Check sheet for the modelled part. Datum: model origin and axes. Units: mm. A direction names the side the tool comes from. Coordinates: 2 decimals unless noted, no trailing zeros. Write each loop counter-clockwise with the first axis right and the second up, starting at its lowest first coordinate (ties: lowest second). Pieces come first, ordered by that corner, then holes. Notation, with made-up numbers: M 60,88 L 117,88 A28 ccw 117,113 Z; hole C 30,64.25 d11. An arc over 180 degrees is marked long. Answer as CSV lines item,"result". Start each with the question number.
1) Section check B-B (y = 63). Record the cut outline in (x, z), and give its area (3 significant figures).
2) Material ranges on L1, parallel to Y at x = 135, z = 45; L2, parallel to Z at x = 498.5, y = -60, recorded low to high. Write a range as [from, to].
3) Access from +Z, -Z, +X, -X, +Y, -Y to the whole of each face (thin tool, end or side, straight path). Record for faces 1 (the flat face through (10, -140, 55)), 2 (the flat face through (-10, 6, 3)).
4) Section check A-A (x = 340.5). Record the cut outline in (y, z), and give its area (3 significant figures).
5) Section check C-C (z = 64.5). Record the cut outline in (x, y), and give its area (3 significant figures).
6) Go/stop test with flat-tipped pins: pin 1 Ø12 at (x, z) = (354, 64) entering from +Y; pin 2 Ø6 at (x, y) = (179.5, -69) entering from +Z. Record where each tip stops, or that it passes through.
Autodesk Inventor part; units mm, degrees
ref_plane "YZ Plane" through (0, 0, 0) normal (1, 0, 0) x (0, 1, 0)
ref_plane "XZ Plane" through (0, 0, 0) normal (0, 1, 0) x (-1, 0, 0)
ref_plane "XY Plane" through (0, 0, 0) normal (0, 0, 1) x (1, 0, 0)
sketch "Sketch1" plane through (0, 0, 0) normal (0, 0, 1) x (1, 0, 0)
  line L0 (700, 140) -> (-700, 140)
  line L1 (-700, 140) -> (-700, -140)
  line L2 (-700, -140) -> (700, -140)
  line L3 (700, -140) -> (700, 140)
  line L4 (700, 140) -> (-700, -140) construction
  line L5 (-700, 140) -> (700, -140) construction
  point P0 (0, 0)
  point P1 (0, 0)
  point P2 (700, 0)
  dimension "d32" = 280
  dimension "d33" = 1400
extrude "Plate1" add sketch "Sketch1" along normal blind 3
sketch "Sketch6" plane through (700, -137, 0) normal (0, -1, 0) x (1, 0, 0)
  line L0 (-1400, 0) -> (0, 0)
  line L1 (0, 0) -> (0, 100)
  line L2 (0, 100) -> (-1400, 100)
  line L3 (-1400, 100) -> (-1400, 0)
edge flange "Flange2" height 100 angle 90 thickness 3 bend radius 5 thickness toward (0, -1, 0) relief round relief width 3 relief depth 1.5 edges at (0, -140, 3) wall of the first edge with corners at (-700, -137, 0) (700, -137, 0) (700, -137, 100) (-700, -137, 100)
bend "Bend2"
corner "Corner2"
sketch "Sketch8" plane through (0, 0, 3) normal (0, 0, 1) x (1, 0, 0)
  line L0 (646.1751, 51.4978) -> (596.1751, 51.4978)
  line L1 (596.1751, 51.4978) -> (596.1751, 101.4978)
  line L2 (596.1751, 101.4978) -> (646.1751, 101.4978)
  line L3 (646.1751, 101.4978) -> (646.1751, 51.4978)
  line L4 (646.1751, 51.4978) -> (596.1751, 101.4978) construction
  line L5 (596.1751, 51.4978) -> (646.1751, 101.4978) construction
  circle A0 centre (652.9949, 44.678) radius 3.5
  circle A1 centre (589.3553, 44.678) radius 3.5
  circle A2 centre (589.3553, 108.3176) radius 3.5
  circle A3 centre (652.9949, 108.3176) radius 3.5
  circle A4 centre (621.1751, 76.4978) radius 45 construction
  point P0 (0, 0)
  dimension "d51" = 50
  dimension "d52" = 50
  dimension "d53" = 7
  dimension "d54" = 90
cut "Cut3" [suppressed]
pattern_linear "Rectangular Pattern1" [suppressed]
equation "\"d55\" = Thickness"
equation "\"d2\" = Thickness"
equation "\"d36\" = BendReliefWidth"
equation "\"d37\" = BendReliefDepth"
equation "\"d38\" = MinimumRemnant"
equation "\"d39\" = TransitionRadius"
equation "\"d42\" = BendRadius"
equation "\"d43\" = CornerReliefSize"
equation "\"d44\" = GapSize"
equation "\"d45\" = JacobiRadiusSize"
equation "\"BendReliefWidth\" = Thickness"
equation "\"BendReliefDepth\" = 0.5 * Thickness"
equation "\"CornerReliefSize\" = 4 * Thickness"
equation "\"MinimumRemnant\" = 2 * Thickness"
equation "\"TransitionRadius\" = BendRadius"
equation "\"JacobiRadiusSize\" = BendRadius"
equation "\"GapSize\" = Thickness"
properties part number "TKS 3006 BOTTOM DS diameter way blind" material "Stainless Steel"
Results found:
1,outline,"M -700,0 L 700,0 L 700,3 L -700,3 Z"
1,area,"4,200 mm2"
2,L1,"y = [-140, -137]"
2,L2,"z = [0, 3]"
3,face 1,"+Z, -Z, +X, -X, -Y"
3,face 2,"+Z, +X, -X, +Y"
4,outline,"M -140,8 A8 ccw -132,0 L 140,0 L 140,3 L -132,3 A5 cw -137,8 L -137,100 L -140,100 Z"
4,area,"1,120 mm2"
5,outline,"M -700,-140 L 700,-140 L 700,-137 L -700,-137 Z"
5,area,"4,200 mm2"
6,pin 1,"stops at y = -137"
6,pin 2,"stops at z = 3"
